Geometry: final body of the model. Coordinates: model frame, mm. A direction names the side the tool comes from. Give positions to 0.01 mm unless a question says otherwise; leave off trailing zeros. Write each loop counter-clockwise with the first axis right and the second up, starting at its lowest first coordinate (ties: lowest second). Pieces come first, ordered by that corner, then holes. Notation, with made-up numbers: (16, 82.25) - (58, 82.25) arc R27 ccw to (58, 101.25) - close; hole circle Ø11 at (23, 6.25). An arc over 180 degrees is marked (long way). Use CSV: the item, a comma, the result in double quotes. Start each with the question number.
(1) Line query: probe 1 along Z at (x, y) = (0, 1.6); probe 2 along X at (y, z) = (0.8, 1.25); probe 3 along Y at (x, z) = (2.75, -2.25). Output: solid intervals per line, ascending. Write a range as [from, to].
(2) First-contact query: pin 1 Ø1 at (x, z) = (2, 2) entering from -Y. Flat tip, straight axial feed; report the tip coordinate or a pass-through.
(3) Section D-D on z = 2. Output: boundary loops of the cut face in (x, y), and give its area (3 significant figures).
(4) Section A-A on x = 0. Output: boundary loops of the cut face in (y, z).
(5) Reachability of faces 1 (the cylindrical face through (3, 2, 0)), 2 (the flat face through (-2, 0, 2)) from +Z, -Z, +X, -X, +Y, -Y: full face, straight path, thin tool, end or side. Return the list, or none.
(6) Section C-C on y = 1.35. Output: boundary loops of the cut face in (x, z).
(7) Section B-B on z = 0. Output: boundary loops of the cut face in (x, y), and give its area (3 significant figures).
(8) Draft query along Z for faces 3 (the cylindrical face through (-3.434, 0.296, -1.081)), 4 (the flat face through (1, 0.6, 3)), 5 (the flat face through (-1, 0.1, -2)), 6 (the cylindrical face through (1.5, 1.23, -0.07)). Return one class per face: released by +Z, released by -Z, zero draft, split by the parting line, or undercut.
Autodesk Inventor part; units mm, degrees
ref_plane "YZ Plane" through (0, 0, 0) normal (1, 0, 0) x (0, 1, 0)
ref_plane "XZ Plane" through (0, 0, 0) normal (0, 1, 0) x (-1, 0, 0)
ref_plane "XY Plane" through (0, 0, 0) normal (0, 0, 1) x (1, 0, 0)
sketch "Sketch1" plane through (0, 0, 0) normal (0, 1, 0) x (-1, 0, 0)
  circle A0 centre (0, 0) radius 3
  circle A1 centre (0, 0) radius 1.5
  circle A2 centre (0, 0) radius 3.6
  circle A3 centre (0, 0) radius 1.9
  circle A4 centre (0, 0) radius 2.6
  dimension "d0" = 6
  dimension "d1" = 3
  dimension "d2" = 7.2
  dimension "d3" = 0.4
  dimension "d4" = 0.4
extrude "Extrusion1" add sketch "Sketch1" along normal blind 2.5 contours A0 | A3 | A4
extrude "Extrusion2" add sketch "Sketch1" along normal blind 0.6 contours A2
extrude "Extrusion3" cut sketch "Sketch1" along normal blind 0.1 contours A4
extrude "Extrusion4" cut sketch "Sketch1" against normal blind 0.1 from surface at 2.5 contours A4
properties part number "Miniatur Flanschkugellager MF 74 ZZ"
Check values:
1,probe 1,"z = [-3, -1.5], [1.5, 3]"
1,probe 2,"x = [-2.73, -0.83], [0.83, 2.73]"
1,probe 3,"y = [0, 0.6]"
2,pin 1,"stops at y = 0"
3,outline,"(-2.99, 0) - (-1.66, 0) - (-1.66, 0.1) - (1.66, 0.1) - (1.66, 0) - (2.99, 0) - (2.99, 0.6) - (2.24, 0.6) - (2.24, 2.5) - (1.66, 2.5) - (1.66, 2.4) - (-1.66, 2.4) - (-1.66, 2.5) - (-2.24, 2.5) - (-2.24, 0.6) - (-2.99, 0.6) - close"
3,area,"11.4 mm²"
4,outline,"(0, -3.6) - (0.6, -3.6) - (0.6, -3) - (2.5, -3) - (2.5, -2.6) - (2.4, -2.6) - (2.4, -1.9) - (2.5, -1.9) - (2.5, -1.5) - (0, -1.5) - (0, -1.9) - (0.1, -1.9) - (0.1, -2.6) - (0, -2.6) - close; (0, 1.5) - (2.5, 1.5) - (2.5, 1.9) - (2.4, 1.9) - (2.4, 2.6) - (2.5, 2.6) - (2.5, 3) - (0.6, 3) - (0.6, 3.6) - (0, 3.6) - (0, 2.6) - (0.1, 2.6) - (0.1, 1.9) - (0, 1.9) - close"
5,face 1,"+Y"
5,face 2,"+Z, -Z, +X, -X, -Y"
6,outline,"circle Ø6 at (0, 0); hole circle Ø3 at (0, 0)"
7,outline,"(-3.6, 0) - (-2.6, 0) - (-2.6, 0.1) - (-1.9, 0.1) - (-1.9, 0) - (-1.5, 0) - (-1.5, 2.5) - (-1.9, 2.5) - (-1.9, 2.4) - (-2.6, 2.4) - (-2.6, 2.5) - (-3, 2.5) - (-3, 0.6) - (-3.6, 0.6) - close; (1.5, 0) - (1.9, 0) - (1.9, 0.1) - (2.6, 0.1) - (2.6, 0) - (3.6, 0) - (3.6, 0.6) - (3, 0.6) - (3, 2.5) - (2.6, 2.5) - (2.6, 2.4) - (1.9, 2.4) - (1.9, 2.5) - (1.5, 2.5) - close"
7,area,"7.94 mm²"
8,face 3,"split by the parting line"
8,face 4,"zero draft"
8,face 5,"undercut"
8,face 6,"undercut"
